Geometry: see drawing. Coordinates: mm, zero at the bounding-box minimum. Coordinates: 2 decimals unless noted, no trailing zeros. Order: outer loops, then holes, each group sorted by start corner. A loop starts at its lowest first (then second) coordinate and runs counter-clockwise, first axis right, second up. Notation, with made-up numbers: (41, -18.5) -> (70, -18.5) arc R9 ccw to (70, -11.5) -> close; hole circle Ø5 at (82, 44). An arc over 180 degrees is marked (long way). Use one line per item in the form item = value.
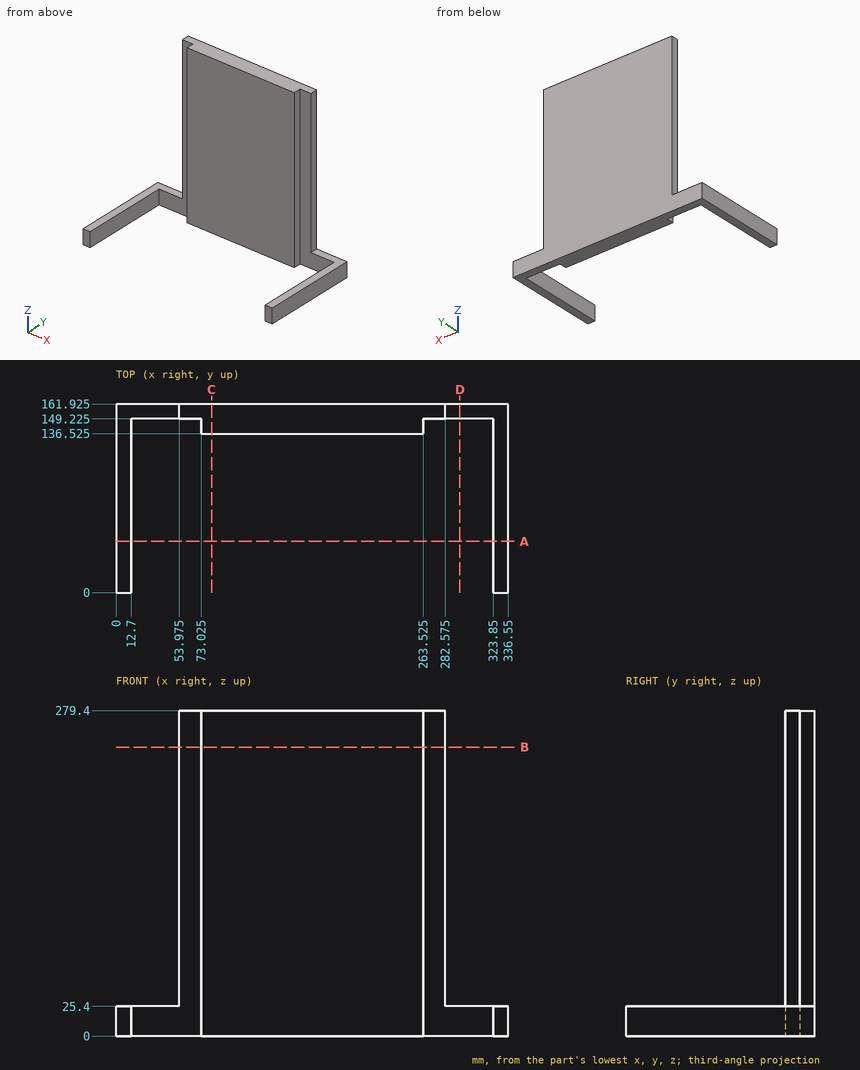
1) Material intervals for probe 1 along Y at (x, z) = (47.5, 17.5) (3 decimals); probe 2 along Y at (x, z) = (177, 129) (3 decimals); probe 3 along X at (y, z) = (144, 72) (3 decimals), sorted ascending. Write a range as from..to.
Results found:
probe_1 = 149.225..161.925
probe_2 = 136.525..161.925
probe_3 = 73.025..263.525
2) Contact query for flat-ended pins moving along their axis: P1, Ø10, axis at y = 158, z = 149, coming from the +X side (3 decimals); P2, Ø12, axis at x = 229.5, z = 51.5, coming from the -Y side (3 decimals); P3, Ø10, axis at y = 143.5, z = 152, coming from the +X side (3 decimals). Output: stop coordinate, or through.
Results found:
P1 = 282.575
P2 = 136.525
P3 = 263.525
3) Section B-B, the plane z = 248. Output: boundary loops of the cut face in (x, y) (3 decimals), and give its area (3 significant figures).
Results found:
outline = (53.975, 149.225) -> (73.025, 149.225) -> (73.025, 136.525) -> (263.525, 136.525) -> (263.525, 149.225) -> (282.575, 149.225) -> (282.575, 161.925) -> (53.975, 161.925) -> close
area = 5,320 mm2
4) Section D-D, the plane x = 295. Output: boundary loops of the cut face in (y, z) (3 decimals).
Results found:
outline = (149.225, 0) -> (161.925, 0) -> (161.925, 25.4) -> (149.225, 25.4) -> close
5) Section C-C, the plane x = 82. Output: boundary loops of the cut face in (y, z) (3 decimals).
Results found:
outline = (136.525, 0) -> (161.925, 0) -> (161.925, 279.4) -> (136.525, 279.4) -> close
6) Section A-A, the plane y = 44. Output: boundary loops of the cut face in (x, z), and give its area (3 significant figures).
Results found:
outline = (0, 0) -> (12.7, 0) -> (12.7, 25.4) -> (0, 25.4) -> close; (323.85, 0) -> (336.55, 0) -> (336.55, 25.4) -> (323.85, 25.4) -> close
area = 645 mm2
